Here's how the part is built. I have some questions about the finished solid (model axes, mm). A direction names the side the tool comes from. Round coordinates to 2 decimals unless told otherwise and drop trailing zeros. Order: outer loops, then holes, each group sorted by start corner. A loop starts at its lowest first (then second) coordinate and runs counter-clockwise, first axis right, second up. Notation, with made-up numbers: M -5.75,0 L 25.25,0 A17 ccw 25.25,8 Z; hole C -19,79.25 d7. An arc over 180 degrees is marked long. Write each question's results on one line, items separated by ' | '. Start each with the question number.
```python
from build123d import *

# Parameters (mm, degrees)
BOSS_EXTRUDE1_DEPTH = 80
SKETCH2_R           = 2.6
CUT_EXTRUDE1_DEPTH  = 325.340177974
SKETCH7_W           = 1.9
SKETCH7_H           = 5.75
CUT_EXTRUDE5_DEPTH  = 5.75
SKETCH9_W           = 10
SKETCH9_H           = 20
CUT_EXTRUDE6_DEPTH  = 2.4
CUT_EXTRUDE7_START  = -9.999995
SKETCH11_R          = 1.75
CUT_EXTRUDE7_DEPTH  = 9.999995
SKETCH13_R          = 3.25
CUT_EXTRUDE8_DEPTH  = 3
SKETCH15_R          = 2.6
BOSS_EXTRUDE7_DEPTH = 80
CUT_EXTRUDE12_DEPTH = 5
SKETCH5_R           = 3.25
CUT_EXTRUDE22_DEPTH = 3
SKETCH30_R          = 1.675
CUT_EXTRUDE23_DEPTH = 25
CUT_EXTRUDE34_DEPTH = 326.347016047
BOSS_EXTRUDE5_DEPTH = 17.5
SKETCH16_W          = 25.561
SKETCH16_H          = 23.4499
SKETCH16_W_2        = 23.8489
CUT_EXTRUDE35_DEPTH = 359.746594886
SKETCH38_W          = 6
SKETCH38_H          = 17.5
CUT_EXTRUDE36_DEPTH = 6
CHAMFER1_SIZE       = 6
CHAMFER2_SIZE       = 6
SKETCH37_R          = 1.6
CUT_EXTRUDE29_DEPTH = 25
BOSS_EXTRUDE8_DEPTH = 30.261


with BuildPart() as part:
    # Sketch1 → Boss-Extrude1 (new body)
    with BuildSketch(Plane.XY):
        Polygon((253.183144434, 132.132101078), (251.183144434, 130.132101078), (251.183144434, 126.632096278), (249.183144434, 124.632096278), (235.948217796, 124.632096278), (233.831644434, 126.74866964), (233.831644434, 140.015512734), (235.948217796, 142.132096278), (311.715071072, 142.132096278), (313.831644434, 140.015522917), (313.831644434, 126.74866964), (311.715071072, 124.632096278), (298.480144434, 124.632096278), (296.480144434, 126.632096278), (296.480144434, 132.132101078), align=None)
    extrude(amount=BOSS_EXTRUDE1_DEPTH)

    # Sketch2 → Cut-Extrude1 (cut, through all)
    with BuildSketch(Plane(origin=(0, 142.132096278, 0), x_dir=(1, 0, 0), z_dir=(0, 1, 0))):
        with Locations(Location((243.081644434, -12.5, 0), (0, 0, 270))):
            Circle(SKETCH2_R)
        with Locations(Location((304.581644434, -40, 0), (0, 0, 270))):
            Circle(SKETCH2_R)
        with Locations(Location((243.081644434, -67.5, 0), (0, 0, 90))):
            Circle(SKETCH2_R)
    extrude(amount=-CUT_EXTRUDE1_DEPTH, mode=Mode.SUBTRACT)

    # Sketch7 → Cut-Extrude5 (cut)
    with BuildSketch(Plane.XZ.offset(-132.132101078)):
        with Locations((290.530144434, 50)):
            Rectangle(SKETCH7_W, SKETCH7_H)
        with Locations((257.133644434, 40)):
            Rectangle(SKETCH7_W, SKETCH7_H)
    extrude(amount=-CUT_EXTRUDE5_DEPTH, mode=Mode.SUBTRACT)

    # Sketch9 → Cut-Extrude6 (cut)
    with BuildSketch(Plane.XZ.offset(-132.132101078)):
        with Locations((273.831644434, 70)):
            Rectangle(SKETCH9_W, SKETCH9_H)
        with Locations((273.831644434, 10)):
            Rectangle(SKETCH9_W, SKETCH9_H)
    extrude(amount=-CUT_EXTRUDE6_DEPTH, mode=Mode.SUBTRACT)

    # Sketch11 → Cut-Extrude7 (cut)
    with BuildSketch(Plane.XZ.offset(-132.132101078).offset(CUT_EXTRUDE7_START)):
        with Locations((263.831644434, 72)):
            Circle(SKETCH11_R)
        with Locations(Location((283.831644434, 72, 0), (0, 0, 180))):
            Circle(SKETCH11_R)
        with Locations((283.831644434, 8)):
            Circle(SKETCH11_R)
        with Locations(Location((263.831644434, 8, 0), (0, 0, 180))):
            Circle(SKETCH11_R)
    extrude(amount=CUT_EXTRUDE7_DEPTH, mode=Mode.SUBTRACT)

    # Sketch13 → Cut-Extrude8 (cut)
    with BuildSketch(Plane(origin=(0, 142.132096278, 0), x_dir=(1, 0, 0), z_dir=(0, 1, 0))):
        with Locations(Location((263.831644434, -8, 0), (0, 0, 270))):
            Circle(SKETCH13_R)
        with Locations(Location((283.831644434, -8, 0), (0, 0, 90))):
            Circle(SKETCH13_R)
        with Locations(Location((283.831644434, -72, 0), (0, 0, 270))):
            Circle(SKETCH13_R)
        with Locations(Location((263.831644434, -72, 0), (0, 0, 90))):
            Circle(SKETCH13_R)
    extrude(amount=-CUT_EXTRUDE8_DEPTH, mode=Mode.SUBTRACT)

    # Sketch15 → Boss-Extrude7 (add, through all)
    with BuildSketch(Plane.ZY.offset(-233.831644434)):
        with BuildLine():
            Line((31.938932188, 142.132096278), (60, 142.132096278))
            Line((60, 142.132096278), (60, 158.122096278))
            ThreePointArc((60, 158.122096278), (56.913417162, 162.741493941), (51.464466094, 161.657630184))
            Line((51.464466094, 161.657630184), (31.938932188, 142.132096278))
        make_face()
        with Locations((55, 158.122096278)):
            Circle(SKETCH15_R, mode=Mode.SUBTRACT)
    extrude(amount=-BOSS_EXTRUDE7_DEPTH)

    # Sketch19 → Cut-Extrude12 (cut)
    with BuildSketch(Plane(origin=(0, 142.132096278, 0), x_dir=(1, 0, 0), z_dir=(0, 1, 0))):
        Polygon((238.260769686, -12.5), (240.67120706, -16.675), (245.492081808, -16.675), (247.902519182, -12.5), (245.492081808, -8.325), (240.67120706, -8.325), align=None)
        Polygon((300.010769686, -40), (302.42120706, -44.175), (307.242081808, -44.175), (309.652519182, -40), (307.242081808, -35.825), (302.42120706, -35.825), align=None)
        Polygon((240.67120706, -71.675), (238.260769686, -67.5), (240.67120706, -63.325), (245.492081808, -63.325), (247.902519182, -67.5), (245.492081808, -71.675), align=None)
    extrude(amount=-CUT_EXTRUDE12_DEPTH, mode=Mode.SUBTRACT)

    # Sketch5 → Cut-Extrude22 (cut)
    with BuildSketch(Plane(origin=(313.831644434, 0, 0), x_dir=(0, 0, -1), z_dir=(1, 0, 0))):
        with Locations(Location((-50, 134.901522917, 0), (0, 0, 90))):
            Circle(SKETCH5_R)
    extrude(amount=-CUT_EXTRUDE22_DEPTH, mode=Mode.SUBTRACT)

    # Sketch30 → Cut-Extrude23 (cut)
    with BuildSketch(Plane(origin=(310.831644434, 0, 0), x_dir=(0, 0, -1), z_dir=(1, 0, 0))):
        with Locations(Location((-50, 134.901522917, 0), (0, 0, 90))):
            Circle(SKETCH30_R)
    extrude(amount=-CUT_EXTRUDE23_DEPTH, mode=Mode.SUBTRACT)

    # Sketch3 → Cut-Extrude34 (cut, through all)
    with BuildSketch(Plane.XZ.offset(-132.132101078)):
        Polygon((296.48017643, 80), (294.98017643, 80), (295.480144434, 17.507999488), (296.480144434, 17.5), align=None)
    extrude(amount=-CUT_EXTRUDE34_DEPTH, mode=Mode.SUBTRACT)

    # Sketch31 → Boss-Extrude5 (add)
    with BuildSketch(Plane(origin=(0, 0, 0), x_dir=(-1, 0, 0), z_dir=(0, 0, -1))):
        Polygon((-296.480144434, 132.132101078), (-296.480144434, 130.132101078), (-294.480144434, 132.132101078), align=None)
    extrude(amount=-BOSS_EXTRUDE5_DEPTH)

    # Sketch16 → Cut-Extrude35 (cut, through all)
    with BuildSketch(Plane.XY.offset(60)):
        with Locations((273.831644434, 153.857046278)):
            Rectangle(SKETCH16_W, SKETCH16_H)
        with Locations((244.426694434, 153.857046278)):
            Rectangle(SKETCH16_W_2, SKETCH16_H)
        with Locations((303.236594434, 153.857046278)):
            Rectangle(SKETCH16_W_2, SKETCH16_H)
    extrude(amount=-CUT_EXTRUDE35_DEPTH, mode=Mode.SUBTRACT)

    # Sketch38 → Cut-Extrude36 (cut)
    with BuildSketch(Plane.ZY.offset(-233.831644434)):
        with Locations((40, 133.382096278)):
            Rectangle(SKETCH38_W, SKETCH38_H)
    extrude(amount=-CUT_EXTRUDE36_DEPTH, mode=Mode.SUBTRACT)

    # Chamfer1
    chamfer1_edges = [part.edges().sort_by_distance(p)[0] for p in [
        (233.831644434, 133.382091187, 43),
    ]]
    chamfer(chamfer1_edges, length=CHAMFER1_SIZE - 0.0001)  # a hair under: the kernel refuses the full size

    # Chamfer2
    chamfer2_edges = [part.edges().sort_by_distance(p)[0] for p in [
        (233.831644434, 133.382091187, 37),
    ]]
    chamfer(chamfer2_edges, length=CHAMFER2_SIZE - 0.0001)  # a hair under: the kernel refuses the full size

    # Sketch37 → Cut-Extrude29 (cut)
    with BuildSketch(Plane.ZY.offset(-239.831644434)):
        with Locations((40, 134.901396278)):
            Circle(SKETCH37_R)
    extrude(amount=-CUT_EXTRUDE29_DEPTH, mode=Mode.SUBTRACT)

    # Sketch39 → Boss-Extrude8 (add)
    with BuildSketch(Plane.ZY.offset(-256.351144434)):
        with BuildLine():
            Line((52.755415069, 152.589963609), (31.938932188, 142.132096278))
            Line((31.938932188, 142.132096278), (60, 142.132096278))
            Line((60, 142.132096278), (60, 148.122096278))
            ThreePointArc((60, 148.122096278), (57.624602384, 152.377852654), (52.755415069, 152.589963609))
        make_face()
    extrude(amount=-BOSS_EXTRUDE8_DEPTH)


solid = part.part
```
(1) I'm going to push flat-ended pins straight in: pin 1 Ø3 at (y, z) = (158.12, 55) entering from -X; pin 2 Ø7 at (x, z) = (263.5, 72.5) entering from +Y; pin 3 Ø5 at (x, y) = (281.5, 155) entering from -Z; pin 4 Ø5 at (x, z) = (283.83, 72) entering from -Y. Where does each tip first touch, or does it pass through?
(2) On a 3-axis mill with a long thin cutter (end or side, diameter ignored), from which of +Z, -Z, +X, -X, +Y, -Y can I reach the whole of each face in a straight line? I mean faces 5 (the cylindrical face through (303.756, 135.802, 51.412)), 6 (the flat face through (264.832, 135, 40)), 7 (the flat face through (233.832, 133, 15)), 8 (the flat face through (246.68, 139.67, 65.38)). Say none if no direction works.
(3) Please list where these lines run through material, in increasing order: line 1 (Y direction, x = 244, z = 40); line 2 (Z direction, x = 307.5, y = 135); line 3 (X direction, y = 129, z = 51).
(4) I want a section at B-B on x = 274. Write out the boundary of the cut face in (y, z).
(5) I want a section at D-D on x = 301. Write out the boundary of the cut face in (y, z) (3 decimals).
(6) If we mould it in two halves opening along X, with no side actions, what happens to faces 1 (the flat face through (252.2, 131.15, 39.44)), 2 (the cylindrical face through (312.353, 137.904, 48.755)), 3 (the cylindrical face through (285.45, 135.68, 7.33)), 4 (the flat face through (285.832, 135, 50))? For each: pulls with the +X half, pulls with the -X half, needs draft (parallel to the pull), parting line crosses it, or undercut.
(7) I want a section at C-C on y = 145. Write out the boundary of the cut face in (x, z), and give its area (3 significant figures).
Solutions:
1) pin 1: through | pin 2: y = 142.13 | pin 3: z = 52.58 | pin 4: y = 132.13
2) face 5: +X | face 6: -X | face 7: +Z, -Z, -X, +Y, -Y | face 8: +Y
3) line 1: 124.63 to 133.3, 136.5 to 142.13 | line 2: 0 to 48.33, 51.67 to 80 | line 3: 233.83 to 251.18, 296.48 to 313.83
4) outline: M 132.13,20 L 134.53,20 L 134.53,0 L 142.13,0 L 142.13,31.94 L 152.59,52.76 A5 ccw 148.12,60 L 142.13,60 L 142.13,80 L 134.53,80 L 134.53,60 L 132.13,60 Z
5) outline: M 124.632,0 L 142.132,0 L 142.132,38.287 L 137.132,38.287 L 137.132,41.713 L 142.132,41.713 L 142.132,80 L 124.632,80 Z; hole C 134.902,50 d3.35
6) face 1: undercut | face 2: needs draft | face 3: undercut | face 4: pulls with the +X half
7) outline: M 256.35,34.81 L 261.05,34.81 L 261.05,37.65 L 286.61,37.65 L 286.61,34.81 L 291.31,34.81 L 291.31,60 L 256.35,60 Z | area: 808 mm^2
